```python
from build123d import *

# Parameters (mm, degrees)
SKETCH_1_R      = 1.5
EXTRUDE_1_DEPTH = 3
SKETCH_2_R      = 1.5
SKETCH_2_R_2    = 0.5
EXTRUDE_2_DEPTH = 3


with BuildPart() as part:
    # 草图1 → 凸台-拉伸1 (new body)
    with BuildSketch(Plane.XY):
        with BuildLine():
            ThreePointArc((31.666666667, 2.494438258), (15, 7.550055679), (-1.666666667, 2.494438258))
            ThreePointArc((-1.666666667, 2.494438258), (-2.494438258, -1.666666667), (1.666666667, -2.494438258))
            ThreePointArc((1.666666667, -2.494438258), (15, 1.550055679), (28.333333333, -2.494438258))
            ThreePointArc((28.333333333, -2.494438258), (32.494438258, -1.666666667), (31.666666667, 2.494438258))
        make_face()
        Circle(SKETCH_1_R, mode=Mode.SUBTRACT)
        with Locations((30, 0)):
            Circle(SKETCH_1_R, mode=Mode.SUBTRACT)
    extrude(amount=EXTRUDE_1_DEPTH)

    # 草图2 → 凸台-拉伸2 (add, through all)
    with BuildSketch(Plane.XY.offset(3)):
        with Locations((30, 0)):
            Circle(SKETCH_2_R)
        with Locations((30, 0)):
            Circle(SKETCH_2_R_2, mode=Mode.SUBTRACT)
    extrude(amount=-EXTRUDE_2_DEPTH)


solid = part.part
```
Check sheet for the modelled part. Datum: model origin and axes. Units: mm. Give positions to 0.01 mm unless a question says otherwise; leave off trailing zeros. Loops run counter-clockwise (first coordinate to the right, second up) from the corner with the lowest first, then second, coordinate; pieces in that order, holes last. Notation, with made-up numbers: M -13.75,33.25 L 5.25,33.25 A24 ccw 5.25,54.25 Z; hole C 24.5,-13.5 d10. An arc over 180 degrees is marked long. Answer in a Markdown table with one row per item.
1) Cross-section at D-D (x = 0.5). Enter the section's corners in (y, z), plus the area to 3 significant figures.
Solutions:
| item | result |
|---|---|
| outline | M -2.96,0 L -1.41,0 L -1.41,3 L -2.96,3 Z; M 1.41,0 L 3.81,0 L 3.81,3 L 1.41,3 Z |
| area | 11.8 mm^2 |
2) Cross-section at B-B (z = 2.2). Enter the section's corners in (x, y), plus the area to 3 significant figures.
Solutions:
| item | result |
|---|---|
| outline | M -1.67,2.49 A3 ccw 1.67,-2.49 A24 cw 28.33,-2.49 A3 ccw 31.67,2.49 A30 ccw Z; hole C 0,0 d3; hole C 30,0 d1 |
| area | 211 mm^2 |
3) Cross-section at C-C (y = 0). Enter the section's corners in (x, z).
Solutions:
| item | result |
|---|---|
| outline | M -3,0 L -1.5,0 L -1.5,3 L -3,3 Z; M 1.5,0 L 6.51,0 L 6.51,3 L 1.5,3 Z; M 23.49,0 L 29.5,0 L 29.5,3 L 23.49,3 Z; M 30.5,0 L 33,0 L 33,3 L 30.5,3 Z |
4) Thickness scan on line 1 (X direction, y = -1.25, z = 2.65); line 2 (Y direction, x = 30, z = 2); line 3 (Y direction, x = 0, z = 1.9). Record the ranges inside material, lowest first.
Solutions:
| item | result |
|---|---|
| line 1 | x = -2.73 to -0.83, 0.83 to 3.75, 26.25 to 32.73 |
| line 2 | y = -3 to -0.5, 0.5 to 3.53 |
| line 3 | y = -3 to -1.5, 1.5 to 3.53 |
5) Cross-section at A-A (x = 30). Enter the section's corners in (y, z).
Solutions:
| item | result |
|---|---|
| outline | M -3,0 L -0.5,0 L -0.5,3 L -3,3 Z; M 0.5,0 L 3.53,0 L 3.53,3 L 0.5,3 Z |
6) Depth check by flat-ended pin: pin 1 (1.5 mm diameter, centred on x = 17.5, y = 0, fed in from -Z). Enter the tip coordinate at first touch or a pass-through.
Solutions:
| item | result |
|---|---|
| pin 1 | passes through |
